Build history of the part. All positions in model axes, mm. Round coordinates to 2 decimals unless told otherwise and drop trailing zeros. Write each loop counter-clockwise with the first axis right and the second up, starting at its lowest first coordinate (ties: lowest second). Pieces come first, ordered by that corner, then holes. Notation, with made-up numbers: (41.5, 34) -> (70.5, 34) arc R18 cw to (70.5, 51) -> close; hole circle Ø9 at (88.5, 5). An arc over 180 degrees is marked (long way). One line per question, with ' | ' between items.
from build123d import *

# Parameters (mm, degrees)
F0_W     = 50.8
F0_H     = 50.8
F1_DEPTH = 50.8
F3_DEPTH = 76.2
F5_DEPTH = 76.2


with BuildPart() as f1:
    # F0 (on Top) → F1 (new body)
    with BuildSketch(Plane.XY):
        Rectangle(F0_W, F0_H)
    extrude(amount=F1_DEPTH)

    # F2 (on face) → F3 (cut)
    with BuildSketch(Plane.XZ.offset(25.4)):
        Polygon((-25.4, 0), (0, 50.8), (-25.4, 50.8), align=None)
    extrude(amount=-F3_DEPTH, mode=Mode.SUBTRACT)

    # F4 (on face) → F5 (cut)
    with BuildSketch(Plane.XZ.offset(25.4)):
        Polygon((25.4, 50.8), (0, 50.8), (25.4, 0), align=None)
    extrude(amount=-F5_DEPTH, mode=Mode.SUBTRACT)


solid = f1.part
(1) Slice it at C-C (y = 11). Write the cut outline in (x, z), then the cut area to 3 significant figures.
Calculated:
outline: (-25.4, 0) -> (25.4, 0) -> (0, 50.8) -> close | area: 1,290 mm2
(2) Wall check: line 1 (X direction, y = -22, z = 48); line 2 (Z direction, x = -23, y = -12.5); line 3 (Z direction, x = 2.5, y = 6.5). Give the ranges that are in metal, low to high. Write a range as from..to.
Calculated:
line 1: -1.4..1.4 | line 2: 0..4.8 | line 3: 0..45.8
(3) Drop flat-ended pins along their axis: pin 1 (6 mm diameter, centred on y = 3, z = 11.5, fed in from +X); pin 2 (4 mm diameter, centred on x = -15.5, y = 12, fed in from +Z); pin 3 (1 mm diameter, centred on y = -4.5, z = 25.5, fed in from -X); pin 4 (5 mm diameter, centred on x = -5.5, z = 42.5, fed in from -Y). Give the stop position or say it passes through.
Calculated:
pin 1: x = 21.15 | pin 2: z = 23.8 | pin 3: x = -12.9 | pin 4: y = -25.4
(4) Slice it at A-A (z = 30.5). Write the cut outline in (x, y), then the cut area to 3 significant figures.
Calculated:
outline: (-10.15, -25.4) -> (10.15, -25.4) -> (10.15, 25.4) -> (-10.15, 25.4) -> close | area: 1,030 mm2
(5) Slice it at B-B (x = -15.5). Write the cut outline in (y, z), then the cut area to 3 significant figures.
Calculated:
outline: (-25.4, 0) -> (25.4, 0) -> (25.4, 19.8) -> (-25.4, 19.8) -> close | area: 1,010 mm2
